from build123d import *

# Parameters (mm, degrees)
CROQUIS1_W                   = 24
CROQUIS1_H                   = 25
CROQUIS1_R                   = 1
SALIENTE_EXTRUIR1_DEPTH      = 1
CROQUIS2_W                   = 8
CROQUIS2_H                   = 8
SALIENTE_EXTRUIR2_DEPTH      = 5.2
CROQUIS3_W                   = 8
CROQUIS3_H                   = 8
CROQUIS3_R                   = 3.5
CORTAR_EXTRUIR1_DEPTH        = 2
CROQUIS4_R                   = 3.5
CROQUIS4_R_2                 = 2.5
CORTAR_EXTRUIR2_DEPTH        = 0.5
SALIENTE_EXTRUIR3_DEPTH      = 3.5
SALIENTE_EXTRUIR3_DEPTH_BACK = 3.5
CROQUIS6_W                   = 5.6
CROQUIS6_H                   = 20
SALIENTE_EXTRUIR4_DEPTH      = 2.8


with BuildPart() as part:
    # Croquis1 → Saliente-Extruir1 (new body)
    with BuildSketch(Plane.XY):
        Rectangle(CROQUIS1_W, CROQUIS1_H)
        with Locations((9.58, -10.5)):
            Circle(CROQUIS1_R, mode=Mode.SUBTRACT)
        with Locations((-2.65, -10.5)):
            Circle(CROQUIS1_R, mode=Mode.SUBTRACT)
        with Locations(Location((9.58, 10.5, 0), (0, 0, 180))):
            Circle(CROQUIS1_R, mode=Mode.SUBTRACT)
        with Locations(Location((-2.65, 10.5, 0), (0, 0, 180))):
            Circle(CROQUIS1_R, mode=Mode.SUBTRACT)
    extrude(amount=SALIENTE_EXTRUIR1_DEPTH)

    # Croquis2 → Saliente-Extruir2 (add)
    with BuildSketch(Plane.XY.offset(1)):
        with Locations((-2.9, 0)):
            Rectangle(CROQUIS2_W, CROQUIS2_H)
    extrude(amount=SALIENTE_EXTRUIR2_DEPTH)

    # Croquis3 → Cortar-Extruir1 (cut)
    with BuildSketch(Plane.XY.offset(6.2)):
        with Locations((-2.9, 0)):
            Rectangle(CROQUIS3_W, CROQUIS3_H)
        with Locations((-2.9, 0)):
            Circle(CROQUIS3_R, mode=Mode.SUBTRACT)
    extrude(amount=-CORTAR_EXTRUIR1_DEPTH, mode=Mode.SUBTRACT)

    # Croquis4 → Cortar-Extruir2 (cut)
    with BuildSketch(Plane.XY.offset(6.2)):
        with Locations((-2.9, 0)):
            Circle(CROQUIS4_R)
        with Locations((-2.9, 0)):
            Circle(CROQUIS4_R_2, mode=Mode.SUBTRACT)
    extrude(amount=-CORTAR_EXTRUIR2_DEPTH, mode=Mode.SUBTRACT)

    # Croquis5 → Saliente-Extruir3 (add, two sides: drawn at the far end of the back side and taken through both)
    with BuildSketch(Plane(origin=(0, 0, 0), x_dir=(1, 0, 0), z_dir=(0, 1, 0)).offset(-SALIENTE_EXTRUIR3_DEPTH_BACK)):
        Polygon((8.58, -1), (6.3, -1), (6.3, -2.2), (9.58, -2.2), (9.58, -1), align=None)
        with BuildLine():
            Line((3.1, -2), (1.1, -2))
            Line((1.1, -2), (1.1, -2.1))
            Line((1.1, -2.1), (3.095012438, -2.1))
            Line((3.095012438, -2.1), (5.095012438, -2.3))
            Line((5.095012438, -2.3), (10.78, -2.3))
            ThreePointArc((10.78, -2.3), (10.83, -2.25), (10.78, -2.2))
            Line((10.78, -2.2), (9.58, -2.2))
            Line((9.58, -2.2), (6.3, -2.2))
            Line((6.3, -2.2), (5.1, -2.2))
            Line((5.1, -2.2), (3.1, -2))
        make_face()
    extrude(amount=SALIENTE_EXTRUIR3_DEPTH + SALIENTE_EXTRUIR3_DEPTH_BACK)

    # Croquis6 → Saliente-Extruir4 (add)
    with BuildSketch(Plane(origin=(0, 0, 0), x_dir=(-1, 0, 0), z_dir=(0, 0, -1))):
        with Locations((9.2, 0)):
            Rectangle(CROQUIS6_W, CROQUIS6_H)
    extrude(amount=SALIENTE_EXTRUIR4_DEPTH)


solid = part.part
Design review of the part built by this model. Coordinates are the model's own, in mm. A direction names the side the tool comes from. Give positions to 0.01 mm unless a question says otherwise; leave off trailing zeros. Loops run counter-clockwise (first coordinate to the right, second up) from the corner with the lowest first, then second, coordinate; pieces in that order, holes last. Notation, with made-up numbers: M -20,-7.75 L -14,-7.75 A26 cw -14,22.25 Z; hole C -26,-9 d1. An arc over 180 degrees is marked long. Answer as a JSON object with one key per item and string values.
Item 1: We need section D-D (x = -2.9). State the section outline as (y, z) points, and give its area (3 significant figures).
Output values:
{"outline": "M -12.5,0 L -11.47,0 L -11.47,1 L -12.5,1 Z; M -9.53,0 L 9.53,0 L 9.53,1 L 4,1 L 4,4.2 L 3.5,4.2 L 3.5,5.7 L 2.5,5.7 L 2.5,6.2 L -2.5,6.2 L -2.5,5.7 L -3.5,5.7 L -3.5,4.2 L -4,4.2 L -4,1 L -9.53,1 Z; M 11.47,0 L 12.5,0 L 12.5,1 L 11.47,1 Z", "area": "59.7 mm2"}
Item 2: Wall thickness on line 1 along X through (y, z) = (10.5, 0.25); line 2 along Y through (x, z) = (9.58, 0.35); line 3 along X through (y, z) = (1.5, 1.75): over which ranges is each line inside the solid? List them lowest first.
Output values:
{"line 1": "x = -12 to -3.65, -1.65 to 8.58, 10.58 to 12", "line 2": "y = -12.5 to -11.5, -9.5 to 9.5, 11.5 to 12.5", "line 3": "x = -6.9 to 1.1, 6.3 to 9.58"}
Item 3: Machinability: for faces 1 (the face through (7, -3.5, 2)), 2 (the face through (8, 0, 2.3)), 3 (the face through (-0.515, 0.751, 5.954)), 4 (the face through (9.58, 0, 2)), which of the approach directions +Z, -Z, +X, -X, +Y, -Y give a long, thin tool a straight path to every point of the face, cutting with its end or side? Answer none if there is none.
Output values:
{"face 1": "+Z, +X, -Y", "face 2": "+Z, +X, +Y, -Y", "face 3": "+Z", "face 4": "+X, +Y, -Y"}
Item 4: We need section A-A (y = -10.5). State the section outline as (x, z) points, and give its area (3 significant figures).
Output values:
{"outline": "M -12,0 L -3.65,0 L -3.65,1 L -12,1 Z; M -1.65,0 L 8.58,0 L 8.58,1 L -1.65,1 Z; M 10.58,0 L 12,0 L 12,1 L 10.58,1 Z", "area": "20.0 mm2"}
Item 5: Mouldability with a two-part tool opening along Y and no side actions: class faces 5 (the face through (-3, -4, 3)), 6 (the face through (-12, 0, -1)), 7 (the face through (7, 3.5, 2)), 8 (the face through (10.12, -9.66, 0.49)) as pulls with the +Y half, pulls with the -Y half, needs draft (parallel to the pull), parting line crosses it, or undercut.
Output values:
{"face 5": "pulls with the -Y half", "face 6": "needs draft", "face 7": "pulls with the +Y half", "face 8": "undercut"}
Item 6: For P1, Ø5, axis at y = 3.5, z = 4, coming from the +X side; P2, Ø2.5, axis at x = 9.58, y = -10.5, coming from the +Z side; P3, Ø1.4, axis at y = 4, z = -1.5, coming from the +X side, all flat-tipped, find the tip position at first contact; note any pin that passes through.
Output values:
{"P1": "stops at x = 10.83", "P2": "stops at z = 1", "P3": "stops at x = -6.4"}
Item 7: We need section B-B (x = 2). State the section outline as (y, z) points.
Output values:
{"outline": "M -12.5,0 L 12.5,0 L 12.5,1 L -12.5,1 Z; M -3.5,2 L 3.5,2 L 3.5,2.1 L -3.5,2.1 Z"}
